Autodesk Inventor part; units mm, degrees
ref_plane "Work Plane1" through (0, 0, 0) normal (0, 1, 0) x (1, 0, 0)
ref_plane "YZ Plane" through (0, 0, 0) normal (1, 0, 0) x (0, 1, 0)
ref_plane "XZ Plane" through (0, 0, 0) normal (0, 1, 0) x (-1, 0, 0)
sketch "Sketch1" plane through (0, 0, 0) normal (1, 0, 0) x (0, 1, 0)
  circle A0 centre (0, 0) radius 6.0706
  circle A1 centre (0, 0) radius 3.2512
  dimension "d0" = 12.1412
  dimension "d1" = 6.5024
extrude "Body" add sketch "Sketch1" along normal blind 0.7112
sketch "Sketch2" plane through (0, 0, 0) normal (-1, 0, 0) x (0, 0, 1)
  circle A0 centre (0, 0) radius 3.2512
  circle A1 centre (0, 0) radius 6.0706
  arc A2 (0.9093, 4.5713) -> (-0.9093, 4.5713) centre (0, 0) ccw
  line L0 (-0.6343, 3.1887) -> (-0.9093, 4.5713)
  line L1 (0, 0) -> (0, 4.6609) construction
  line L2 (0.6343, 3.1887) -> (0.9093, 4.5713)
  line L3 (-0.6343, 3.1887) -> (0, 0) construction
  line L4 (0.6343, 3.1887) -> (0, 0) construction
  dimension "d4" = 9.3218
  dimension "d5" = 11.25
extrude "Cut" cut sketch "Sketch2" against normal blind 0.7112 contours A0 L0 A2 L2
fillet "Fillet1" radius 0.1951 2 edges at (0.3556, 4.5713, 0.9093) (0.3556, 4.5713, -0.9093)
pattern_circular "Cuts" count 8 over 360 about axis through (-10, 0, 0) along (1, 0, 0) of "Cut", "Fillet1"
ref_plane "Work Plane1" through (0, 0, 0) normal (0, 1, 0) x (1, 0, 0)
equation "\"d0\" = SD2"
equation "\"d1\" = SD1"
equation "\"d2\" = SD"
equation "\"d4\" = 0.5 * SD2 + 0.5 * SD1"
equation "\"d6\" = SD"
equation "\"d8\" = 0.03 * SD1"
equation "\"SD1\" = 6.5024"
equation "\"SD2\" = 12.1412"
equation "\"SD\" = 0.7112"
equation "\"NND\" = 6.35"
properties part number "ASME B18.21.1 - 1/4. Carbon Steel" material "Steel, Mild"
Could you check a few things on this model? Use its own coordinates, in mm. A direction names the side the tool comes from. Give positions to 0.01 mm unless a question says otherwise; leave off trailing zeros. Order: outer loops, then holes, each group sorted by start corner. A loop starts at its lowest first (then second) coordinate and runs counter-clockwise, first axis right, second up. Notation, with made-up numbers: (40, 35.5) - (65, 35.5) arc R19 ccw to (65, 64.5) - close; hole circle Ø7 at (-26.75, 67.25). An arc over 180 degrees is marked (long way). One line per item, written item: value. Start each with the question number.
1. Imagine slicing it at C-C on z = -3. List the corners of the cut face in (x, y) for me, plus the area to 3 significant figures.
2. If I drill on probe 1 along Z at (x, y) = (0.35, 0); probe 2 along Y at (x, z) = (0.1, -3.5); probe 3 along Y at (x, z) = (0.4, -0.5), over which ranges is the centre line in solid material (lowest first)?
3. For faces 4 (the face through (0, 4, -1)), 5 (the face through (0.35, 3.29, 3.3)), which set-ups out of +Z, -Z, +X, -X, +Y, -Y let a thin tool reach every point of the face, with its end or its side?
4. Imagine slicing it at A-A on y = 0. List the corners of the cut face in (x, z) for me.
5. Thinking about a two-plate mould opening in Z: for faces 1 (the face through (0.35, 3.3, -3.29)), 2 (the face through (0.711, 4, -1)), 3 (the face through (0.351, -1.316, 5.926)), which applies, +Z half, -Z half, draft (parallel to the pull), parting line (faces both ways), or undercut?
Values:
1. outline: (0, -5.28) - (0.71, -5.28) - (0.71, -3.57) - (0, -3.57) - close; (0, -2) - (0.71, -2) - (0.71, -1.25) - (0, -1.25) - close; (0, 1.25) - (0.71, 1.25) - (0.71, 2) - (0, 2) - close; (0, 3.57) - (0.71, 3.57) - (0.71, 5.28) - (0, 5.28) - close
1. area: 3.50 mm²
2. probe 1: -6.07 to -4.66, 4.66 to 6.07
2. probe 2: -4.96 to -3.08, -2.34 to -0.7, 0.7 to 2.34, 3.08 to 4.96
2. probe 3: -6.05 to -4.63, 4.63 to 6.05
3. face 4: +Z, -Z, -X, +Y, -Y
3. face 5: +X, -X
4. outline: (0, -6.07) - (0.71, -6.07) - (0.71, -4.66) - (0, -4.66) - close; (0, 4.66) - (0.71, 4.66) - (0.71, 6.07) - (0, 6.07) - close
5. face 1: undercut
5. face 2: draft
5. face 3: parting line
